Geometry: final body of the model. Coordinates: model frame, mm. A direction names the side the tool comes from. Give positions to 0.01 mm unless a question says otherwise; leave off trailing zeros. Loops run counter-clockwise (first coordinate to the right, second up) from the corner with the lowest first, then second, coordinate; pieces in that order, holes last. Notation, with made-up numbers: (74.25, -39.5) - (79.25, -39.5) arc R23 cw to (79.25, -24.5) - close; hole circle Ø4 at (74.25, 4). An arc over 180 degrees is marked (long way). Use CSV: the item, a comma, the result in double quotes. Start each with the question number.
```python
from build123d import *

# Parameters (mm, degrees)
SKETCH_1_W          = 50
SKETCH_1_H          = 68
EXTRUDE_1_DEPTH     = 3
FILLET_1_R          = 2
SKETCH_1_5_R        = 0.5
CUT_EXTRUDE_1_DEPTH = 43.308391603
SKETCH_1_6_W        = 43
SKETCH_1_6_H        = 61
CUT_EXTRUDE_2_DEPTH = 1.5
CHAMFER_1_SIZE      = 0.376
CUT_EXTRUDE_3_DEPTH = 43.308391603
SKETCH_6_W          = 14
SKETCH_6_H          = 7
CUT_EXTRUDE_4_DEPTH = 2
SKETCH_6_3_W        = 6.5
SKETCH_6_3_H        = 6.5
CUT_EXTRUDE_5_DEPTH = 43.308391603
FILLET_2_R          = 0.6


with BuildPart() as part:
    # 草图1 → 凸台-拉伸1 (new body)
    with BuildSketch(Plane.XY):
        Rectangle(SKETCH_1_W, SKETCH_1_H)
    extrude(amount=EXTRUDE_1_DEPTH)

    # 圆角1
    fillet_1_edges = [part.edges().sort_by_distance(p)[0] for p in [
        (-25, -34, 1.5),
        (-25, 34, 1.5),
        (25, 34, 1.5),
        (25, -34, 1.5),
    ]]
    fillet(fillet_1_edges, radius=FILLET_1_R)

    # 草图1<5> → 切除-拉伸1 (cut, through all)
    with BuildSketch(Plane.XY):
        with Locations((23, 32)):
            Circle(SKETCH_1_5_R)
        with Locations((-23, 32)):
            Circle(SKETCH_1_5_R)
        with Locations((-23, -32)):
            Circle(SKETCH_1_5_R)
        with Locations((23, -32)):
            Circle(SKETCH_1_5_R)
    extrude(amount=CUT_EXTRUDE_1_DEPTH, mode=Mode.SUBTRACT)

    # 草图1<6> → 切除-拉伸2 (cut)
    with BuildSketch(Plane.XY):
        Rectangle(SKETCH_1_6_W, SKETCH_1_6_H)
    extrude(amount=CUT_EXTRUDE_2_DEPTH, mode=Mode.SUBTRACT)

    # 倒角1
    chamfer_1_edges = [part.edges().sort_by_distance(p)[0] for p in [
        (22.5, -32, 3),
        (-23.5, -32, 3),
        (-23.5, 32, 3),
        (22.5, 32, 3),
    ]]
    chamfer(chamfer_1_edges, length=CHAMFER_1_SIZE)

    # 草图5 → 切除-拉伸3 (cut, through all)
    with BuildSketch(Plane.XY.offset(3)):
        with BuildLine():
            Line((15.357692994, -4.714172352), (16.090307006, -4.714172352))
            ThreePointArc((16.090307006, -4.714172352), (17.009545821, -4.333411167), (17.390307006, -3.414172352))
            Line((17.390307006, -3.414172352), (17.390307006, 3.414172352))
            ThreePointArc((17.390307006, 3.414172352), (17.009545821, 4.333411167), (16.090307006, 4.714172352))
            Line((16.090307006, 4.714172352), (15.357692994, 4.714172352))
            ThreePointArc((15.357692994, 4.714172352), (14.438454179, 4.333411167), (14.057692994, 3.414172352))
            Line((14.057692994, 3.414172352), (14.057692994, -3.414172352))
            ThreePointArc((14.057692994, -3.414172352), (14.438454179, -4.333411167), (15.357692994, -4.714172352))
        make_face()
    extrude(amount=-CUT_EXTRUDE_3_DEPTH, mode=Mode.SUBTRACT)

    # 草图6 → 切除-拉伸4 (cut)
    with BuildSketch(Plane.XY):
        with Locations((0, 15)):
            Rectangle(SKETCH_6_W, SKETCH_6_H)
    extrude(amount=CUT_EXTRUDE_4_DEPTH, mode=Mode.SUBTRACT)

    # 草图6<3> → 切除-拉伸5 (cut, through all)
    with BuildSketch(Plane.XY):
        with Locations((-14, -16.5)):
            Rectangle(SKETCH_6_3_W, SKETCH_6_3_H)
    extrude(amount=CUT_EXTRUDE_5_DEPTH, mode=Mode.SUBTRACT)

    # 圆角2
    fillet_2_edges = [part.edges().sort_by_distance(p)[0] for p in [
        (0, -34, 3),
        (-25, 0, 3),
        (25, 0, 3),
        (0, 34, 3),
        (-24.414213562, 33.414213562, 3),
        (24.414213562, 33.414213562, 3),
        (24.414213562, -33.414213562, 3),
        (-24.414213562, -33.414213562, 3),
    ]]
    fillet(fillet_2_edges, radius=FILLET_2_R)


solid = part.part
```
Item 1: Section B-B (x = -5.5). Output: boundary loops of the cut face in (y, z), plus the area to 3 significant figures.
Item 2: Section A-A (y = -15). Output: boundary loops of the cut face in (x, z).
Item 3: Reachability of faces 4 (the flat face through (0, 0, 1.5)), 5 (the cylindrical face through (-24.43, 33.4, 1.22)), 6 (the flat face through (-14, -13.25, 2)) from +Z, -Z, +X, -X, +Y, -Y: full face, straight path, thin tool, end or side. Return the list, or none.
Item 4: Pin query (flat end, axial travel): pin 1 Ø1.5 at (x, y) = (13, -7) entering from -Z; pin 2 Ø3.5 at (x, y) = (-1, 14) entering from -Z. Return the tip coordinate at first contact, or that it passes through.
Item 5: Mould query, pull axis X, two halves, no side actions, for faces 1 (the flat face through (-10.75, -17, 2)), 2 (the flat face through (-25, 0, 1)), 3 (the cylindrical face through (24.43, 33.4, 1.22)). Classes: pulls with the +X half, pulls with the -X half, needs draft (parallel to the pull), parting line crosses it, or undercut.
Item 6: Section C-C (y = 9). Output: boundary loops of the cut face in (x, z).
Item 7: Ray query, probe 1 along Y at (x, z) = (-23, 0.95); probe 2 along X at (y, z) = (32, 1.55); probe 3 along Y at (x, z) = (16, 0.9). Return the intervals inside material, ascending.
Outcome:
1,outline,"(-34, 0) - (-30.5, 0) - (-30.5, 1.5) - (11.5, 1.5) - (11.5, 2) - (18.5, 2) - (18.5, 1.5) - (30.5, 1.5) - (30.5, 0) - (34, 0) - (34, 2.4) arc R0.6 ccw to (33.4, 3) - (-33.4, 3) arc R0.6 ccw to (-34, 2.4) - close"
1,area,"109 mm2"
2,outline,"(-25, 0) - (-21.5, 0) - (-21.5, 1.5) - (-17.25, 1.5) - (-17.25, 3) - (-24.4, 3) arc R0.6 ccw to (-25, 2.4) - close; (-10.75, 1.5) - (21.5, 1.5) - (21.5, 0) - (25, 0) - (25, 2.4) arc R0.6 ccw to (24.4, 3) - (-10.75, 3) - close"
3,face 4,"-Z"
3,face 5,"+Z, -Z, -X, +Y"
3,face 6,"+Z, -Z"
4,pin 1,"stops at z = 1.5"
4,pin 2,"stops at z = 2"
5,face 1,"undercut"
5,face 2,"pulls with the -X half"
5,face 3,"pulls with the +X half"
6,outline,"(-25, 0) - (-21.5, 0) - (-21.5, 1.5) - (21.5, 1.5) - (21.5, 0) - (25, 0) - (25, 2.4) arc R0.6 ccw to (24.4, 3) - (-24.4, 3) arc R0.6 ccw to (-25, 2.4) - close"
7,probe 1,"y = -34 to -32.5, -31.5 to 31.5, 32.5 to 34"
7,probe 2,"x = -25 to -23.5, -22.5 to 22.5, 23.5 to 25"
7,probe 3,"y = -34 to -30.5, 30.5 to 34"
